Could you check a few things on this model? Use its own coordinates, in mm. A direction names the side the tool comes from. Round coordinates to 2 decimals unless told otherwise and drop trailing zeros. Loops run counter-clockwise (first coordinate to the right, second up) from the corner with the lowest first, then second, coordinate; pieces in that order, holes last. Notation, with made-up numbers: (76.25, -9.5) -> (119.25, -9.5) arc R24 ccw to (119.25, 10.5) -> close; hole circle Ø9 at (2.5, 71.5). An arc over 180 degrees is marked (long way). Put each result on its own line as item: value. Start each with the question number.
1. Imagine slicing it at B-B, the plane z = 3.5. Please give me the cut outline in (x, y).
2. Imagine slicing it at D-D, the plane y = -18.57. Please give me the cut outline in (x, z).
3. Imagine slicing it at A-A, the plane y = -2.5. Please give me the cut outline in (x, z).
4. If we mould it in two halves opening along X, with no side actions, what happens to faces 4 (the flat face through (22.8, -14, 0)), 5 (the cylindrical face through (8.05, 1.52, -33.58)), 6 (the flat face through (22, 7, -26.05))? For each: pulls with the +X half, pulls with the -X half, needs draft (parallel to the pull), parting line crosses it, or undercut.
5. Imagine slicing it at C-C, the plane x = 6. Please give me the cut outline in (y, z), and give its area (3 significant figures).
6. I need wall thicknesses on line 1 (Z direction, x = 11, y = 5); line 2 (X direction, y = 1, z = 0.5); line 3 (Z direction, x = 19, y = 3.5). Which ranges of each line are inside material? Lowest first, please. Write a range as [from, to].
7. Which directions (+Z, -Z, +X, -X, +Y, -Y) give clear straight access to the entire face, cutting with the end or side of a thin tool? Please do faces 1 (the flat face through (17, 9, -16.05)), 2 (the cylindrical face through (7.511, -17.185, -33.585)), 3 (the flat face through (12, 0, -15)).
8. I'm going to push flat-ended pins straight in: P1, Ø3.5, axis at x = 24, z = -2, coming from the +Y side; P2, Ø2.5, axis at x = 6, y = 1.43, coming from the -Z side; P3, Ø1.5, axis at y = -8.5, z = -9, coming from the -X side; P4, Ø2, axis at y = 9.5, z = -7, coming from the +X side. Where does each tip first touch, or does it pass through?
```python
from build123d import *

# Parameters (mm, degrees)
SKETCH1_R                = 0.85
BOSS_EXTRUDE1_DEPTH      = 7
BOSS_EXTRUDE2_DEPTH      = 11.2
BOSS_EXTRUDE2_DEPTH_BACK = 7
SKETCH3_W                = 11
SKETCH3_H                = 11.2
CUT_EXTRUDE1_DEPTH       = 42
SKETCH4_W                = 10
SKETCH4_H                = 32.1
BOSS_EXTRUDE3_DEPTH      = 5
SKETCH5_W                = 7
SKETCH5_H                = 6
BOSS_EXTRUDE4_DEPTH      = 32.1
SKETCH6_W                = 32.8
SKETCH6_H                = 7
BOSS_EXTRUDE5_DEPTH      = 10
SKETCH8_W                = 10
SKETCH8_H                = 7
BOSS_EXTRUDE7_DEPTH      = 32.8
CHAMFER2_SIZE            = 1
CHAMFER3_SIZE            = 3
CHAMFER4_SIZE            = 3
CHAMFER8_SIZE            = 0.5
CHAMFER9_SIZE            = 1
SKETCH13_W               = 12
SKETCH13_H               = 45.14
BOSS_EXTRUDE10_DEPTH     = 10
SKETCH14_R               = 2.05
CUT_EXTRUDE2_DEPTH       = 5
SKETCH15_W               = 7
SKETCH15_H               = 0.25
CUT_EXTRUDE3_DEPTH       = 39


with BuildPart() as part:
    # Sketch1 → Boss-Extrude1 (new body)
    with BuildSketch(Plane(origin=(0, 0, 0), x_dir=(1, 0, 0), z_dir=(0, 1, 0))):
        Polygon((0, -16.05), (0, 16.05), (17, 16.05), (17, 11.25), (5, 11.25), (5, -11.25), (17, -11.25), (17, -16.05), align=None)
        with Locations((11, 13.65)):
            Circle(SKETCH1_R, mode=Mode.SUBTRACT)
        with Locations((11, -13.65)):
            Circle(SKETCH1_R, mode=Mode.SUBTRACT)
    extrude(amount=BOSS_EXTRUDE1_DEPTH)

    # Sketch2 → Boss-Extrude2 (add, two sides)
    with BuildSketch(Plane.XZ) as boss_extrude2_sk:
        Polygon((17, 11.25), (27.8, 11.25), (27.8, -11.25), (17, -11.25), (17, -16.05), (32.8, -16.05), (32.8, 16.05), (17, 16.05), align=None)
    extrude(amount=BOSS_EXTRUDE2_DEPTH)
    extrude(boss_extrude2_sk.sketch, amount=-BOSS_EXTRUDE2_DEPTH_BACK)

    # Sketch3 → Cut-Extrude1 (cut)
    with BuildSketch(Plane.XY.offset(16.05)):
        with Locations((22.5, -5.6)):
            Rectangle(SKETCH3_W, SKETCH3_H)
    extrude(amount=-CUT_EXTRUDE1_DEPTH, mode=Mode.SUBTRACT)

    # Sketch4 → Boss-Extrude3 (add)
    with BuildSketch(Plane.XZ.offset(11.2)):
        with Locations((27.8, 0)):
            Rectangle(SKETCH4_W, SKETCH4_H)
    extrude(amount=BOSS_EXTRUDE3_DEPTH)

    # Sketch5 → Boss-Extrude4 (add)
    with BuildSketch(Plane.XY.offset(16.05)):
        with Locations((24.5, -3)):
            Rectangle(SKETCH5_W, SKETCH5_H)
    extrude(amount=-BOSS_EXTRUDE4_DEPTH)



with BuildPart() as body_2:
    # Sketch6 → Boss-Extrude5 (new body)
    with BuildSketch(Plane(origin=(0, 0, -16.05), x_dir=(-1, 0, 0), z_dir=(0, 0, -1))):
        with Locations((-16.4, 10.5)):
            Rectangle(SKETCH6_W, SKETCH6_H)
    extrude(amount=BOSS_EXTRUDE5_DEPTH)


with BuildPart() as part_1:
    add(part.part)

    add(body_2.part)  # Boss-Extrude7 merges body 2
    # Sketch8 → Boss-Extrude7 (add)
    with BuildSketch(Plane.ZY):
        with Locations((-21.05, 3.5)):
            Rectangle(SKETCH8_W, SKETCH8_H)
    extrude(amount=-BOSS_EXTRUDE7_DEPTH)

    # Chamfer2
    chamfer2_edges = [part_1.edges().sort_by_distance(p)[0] for p in [
        (26.9, 0, -16.05),
    ]]
    chamfer(chamfer2_edges, length=CHAMFER2_SIZE)

    # Chamfer3
    chamfer3_edges = [part_1.edges().sort_by_distance(p)[0] for p in [
        (0, 3.5, 16.05),
        (32.8, -4.6, 16.05),
    ]]
    chamfer(chamfer3_edges, length=CHAMFER3_SIZE)

    # Chamfer4
    chamfer4_edges = [part_1.edges().sort_by_distance(p)[0] for p in [
        (16.4, 14, -16.05),
    ]]
    chamfer(chamfer4_edges, length=CHAMFER4_SIZE)

    # Chamfer8
    chamfer8_edges = [part_1.edges().sort_by_distance(p)[0] for p in [
        (32.8, 0, -21.55),
        (32.8, -8.6, -16.05),
        (32.8, -0.5, -16.55),
        (27.8, -16.2, -16.05),
    ]]
    chamfer(chamfer8_edges, length=CHAMFER8_SIZE)

    # Chamfer9
    chamfer9_edges = [part_1.edges().sort_by_distance(p)[0] for p in [
        (21, 0, -13.65),
        (21, 0, 13.65),
    ]]
    chamfer(chamfer9_edges, length=CHAMFER9_SIZE)

    # Sketch13 → Boss-Extrude10 (add)
    with BuildSketch(Plane(origin=(0, 0, -26.05), x_dir=(-1, 0, 0), z_dir=(0, 0, -1))):
        with Locations((-6, -8.57)):
            Rectangle(SKETCH13_W, SKETCH13_H)
    extrude(amount=BOSS_EXTRUDE10_DEPTH)

    # Sketch14 → Cut-Extrude2 (cut)
    with BuildSketch(Plane(origin=(0, 0, -36.05), x_dir=(-1, 0, 0), z_dir=(0, 0, -1))):
        with Locations((-6, 1.43)):
            Circle(SKETCH14_R)
        with Locations((-6, -18.57)):
            Circle(SKETCH14_R)
    extrude(amount=-CUT_EXTRUDE2_DEPTH, mode=Mode.SUBTRACT)

    # Sketch15 → Cut-Extrude3 (cut)
    with BuildSketch(Plane.XY.offset(16.05)):
        with Locations((24.5, -11.325)):
            Rectangle(SKETCH15_W, SKETCH15_H)
        with Locations((24.5, -5.875)):
            Rectangle(SKETCH15_W, SKETCH15_H)
    extrude(amount=-CUT_EXTRUDE3_DEPTH, mode=Mode.SUBTRACT)


solid = part_1.part
```
Entries:
1. outline: (0, 0) -> (5, 0) -> (5, 7) -> (0, 7) -> close; (21, -5.75) -> (28, -5.75) -> (28, -11.45) -> (22.8, -11.45) -> (22.8, -16.2) -> (32.8, -16.2) -> (32.8, 7) -> (27.8, 7) -> (27.8, 0) -> (21, 0) -> close
2. outline: (0, -36.05) -> (3.95, -36.05) -> (3.95, -31.05) -> (8.05, -31.05) -> (8.05, -36.05) -> (12, -36.05) -> (12, -26.05) -> (0, -26.05) -> close
3. outline: (0, -36.05) -> (12, -36.05) -> (12, -26.05) -> (0, -26.05) -> close; (21, -16.05) -> (32.3, -16.05) -> (32.8, -15.55) -> (32.8, 13.05) -> (29.8, 16.05) -> (21, 16.05) -> close
4. face 4: pulls with the -X half
4. face 5: undercut
4. face 6: needs draft
5. outline: (-31.14, -36.05) -> (-20.62, -36.05) -> (-20.62, -31.05) -> (-16.52, -31.05) -> (-16.52, -36.05) -> (-0.62, -36.05) -> (-0.62, -31.05) -> (3.48, -31.05) -> (3.48, -36.05) -> (14, -36.05) -> (14, -19.05) -> (11, -16.05) -> (7, -16.05) -> (7, -11.25) -> (0, -11.25) -> (0, -26.05) -> (-31.14, -26.05) -> close; (0, 11.25) -> (7, 11.25) -> (7, 16.05) -> (0, 16.05) -> close
5. area: 613 mm^2
6. line 1: [-36.05, -14.5], [-12.8, -11.25], [11.25, 12.8], [14.5, 16.05]
6. line 2: [0, 5], [27.8, 32.8]
6. line 3: [-26.05, -11.25], [11.25, 16.05]
7. face 1: +Z, +X, -X, +Y
7. face 2: -Z
7. face 3: -X, -Y
8. P1: y = 0
8. P2: z = -31.05
8. P3: x = 28
8. P4: through
